from build123d import *

# Parameters (mm, degrees)
F3_R = 0.254


# Not quite as in the source:
# - a fillet or chamfer that OpenCascade refuses, or shapes differently, is made with other operations: its cross-section is extruded or revolved along the edge and cut away or added


with BuildPart() as f1:
    # F0 (on Top) → F1 (revolve)
    with BuildSketch(Plane.XY):
        Polygon((-70.4, 0), (0, 0), (0, 23), (-4.4, 23), (-6.7094010768, 19), (-10.0905989232, 19), (-12.4, 23), (-20, 23), (-20, 14.875), (-22, 14.875), (-22, 15.875), (-70.4, 8.815), align=None)
    revolve(axis=Axis((-35.2, 0, 0), (1, 0, 0)))

    # F2: chamfer of 0.381 on 3 edges, made by hand

    # F2_s1 → F2_t2 (revolve, cut)
    with BuildSketch(Plane.XY):
        Polygon((0, 22.619), (-0.381, 23), (0, 23), align=None)
    revolve(axis=Axis((0, 0, 0), (1, 0, 0)), mode=Mode.SUBTRACT)

    # F2_s3 → F2_t4 (revolve, cut)
    with BuildSketch(Plane.XY):
        Polygon((-19.619, 23), (-20, 22.619), (-20, 23), align=None)
    revolve(axis=Axis((-20, 0, 0), (1, 0, 0)), mode=Mode.SUBTRACT)

    # F2_s5 → F2_t6 (revolve, cut)
    with BuildSketch(Plane.XY):
        Polygon((-70.4, 8.4855436088), (-70.0739936383, 8.8625538205), (-70.4, 8.815), align=None)
    revolve(axis=Axis((-70.4, 0, 0), (1, 0, 0)), mode=Mode.SUBTRACT)

    # F3
    f3_edges = [f1.edges().sort_by_distance(p)[0] for p in [
        (-22, -15.875, 0),
        (-22, -14.875, 0),
        (-20, -14.875, 0),
    ]]
    fillet(f3_edges, radius=F3_R)


solid = f1.part
For this review, take the finished solid that the model builds, in its own axes (mm). A direction names the side the tool comes from. Coordinates: 2 decimals unless noted, no trailing zeros. Loops run counter-clockwise (first coordinate to the right, second up) from the corner with the lowest first, then second, coordinate; pieces in that order, holes last. Notation, with made-up numbers: (-21, 89.25) - (16, 89.25) arc R20 ccw to (16, 125.25) - close; hole circle Ø6 at (48, 78.5). An arc over 180 degrees is marked (long way). Return JSON: item names as keys, results as strings.
Item 1: Take a section at C-C (x = -57). Give the boundary of the cut face in (y, z), then the cut area to 3 significant figures.
Determined:
{"outline": "circle Ø21.54 at (0, 0)", "area": "364 mm2"}
Item 2: For faces 1 (the flat face through (-20, 5, -15)), 2 (the cylindrical face through (-16.06, -2.994, 22.804)), list the 3-axis set-ups (+Z, -Z, +X, -X, +Y, -Y) from which the entire face can be reached by the end or side of a thin tool; tool diameter is ignored.
Determined:
{"face 1": "none", "face 2": "+X, -X"}
Item 3: For line 1 (X direction, y = -17, z = 4); line 2 (X direction, y = -15.5, z = 13); line 3 (X direction, y = -17, z = 12.5), list the stretches that pass through material, from the lowest coordinate up.
Determined:
{"line 1": "x = -20 to 0", "line 2": "x = -20 to -10.8, -6 to 0", "line 3": "x = -20 to -11.3, -5.5 to 0"}
Item 4: Mouldability with a two-part tool opening along X and no side actions: class faces 3 (the conical face through (-10.235, 8.883, -17.078)), 4 (the cylindrical face through (-2.419, -2.994, 22.804)), 5 (the flat face through (-70.4, 0, 0)) as pulls with the +X half, pulls with the -X half, needs draft (parallel to the pull), parting line crosses it, or undercut.
Determined:
{"face 3": "undercut", "face 4": "needs draft", "face 5": "pulls with the -X half"}
Item 5: Insertion check: pin 1 (6 mm diameter, centred on x = -46, z = 11.5, fed in from -Y); pin 2 (12 mm diameter, centred on x = -30.5, z = 9.5, fed in from -Y); pin 3 (1.5 mm diameter, centred on x = -62.5, y = 3.5, fed in from -Z). Each pin has a flat end and moves straight along its axis. Give the tip position at first contact, or say it passes through.
Determined:
{"pin 1": "stops at y = -9.06", "pin 2": "stops at y = -14.45", "pin 3": "stops at z = -9.61"}
Item 6: Take a section at D-D (x = -25). Give the boundary of the cut face in (y, z).
Determined:
{"outline": "circle Ø30.87 at (0, 0)"}
